Answer from the drawing. Dimensions are ordinates in mm from the lowest x, y and z of the part. A direction names the side the tool comes from. Coordinates: 2 decimals unless noted, no trailing zeros. Write each loop counter-clockwise with the first axis right and the second up, starting at its lowest first coordinate (ties: lowest second). Pieces come first, ordered by that corner, then holes. Notation, with made-up numbers: (49, 33.25) -> (68, 33.25) arc R20 cw to (68, 49.25) -> close; hole circle Ø1 at (54.25, -31.5). An arc over 180 degrees is marked (long way). Answer as a JSON object with one key per item and string values. Group by question number.
(1) Find section D-D (y = 4.5). Give the vertices of the cut face in (x, z).
(2) Flat-ended cylindrical pins translate along their axes: P1, Ø3, axis at y = 11.5, z = 4.5, coming from the -X side; P2, Ø1.5, axis at x = 16.5, z = 0.5, coming from the +Y side; P3, Ø1.2, axis at x = 17.5, z = 3, coming from the -Y side. Find the tip coordinate at first contact, or state that the pin passes through.
(3) For a pull along X with two mould halves and no side action, classify the marked faces 3, 4, 5 and 6 as +X half, -X half, draft (parallel to the pull), parting line (faces both ways), or undercut.
(4) Find section B-B (y = 10). Give the vertices of the cut face in (x, z) (1 decimal).
(5) Straight lines are drawn through the part: L1, parallel to Y at x = 10.5, z = 2.7; L2, parallel to X at y = 1.9, z = 2.95; L3, parallel to X at y = 10.75, z = 2. For each, find the intervals that lie inside material, in ascending order.
(6) Find section A-A (z = 0.9). Give the vertices of the cut face in (x, y).
(7) Find section C-C (x = 16.5). Give the vertices of the cut face in (y, z).
(8) Which of the six approach directions +Z, -Z, +X, -X, +Y, -Y give full straight-line access (tool end or side, diameter ignored) to the marked faces 1 and 2?
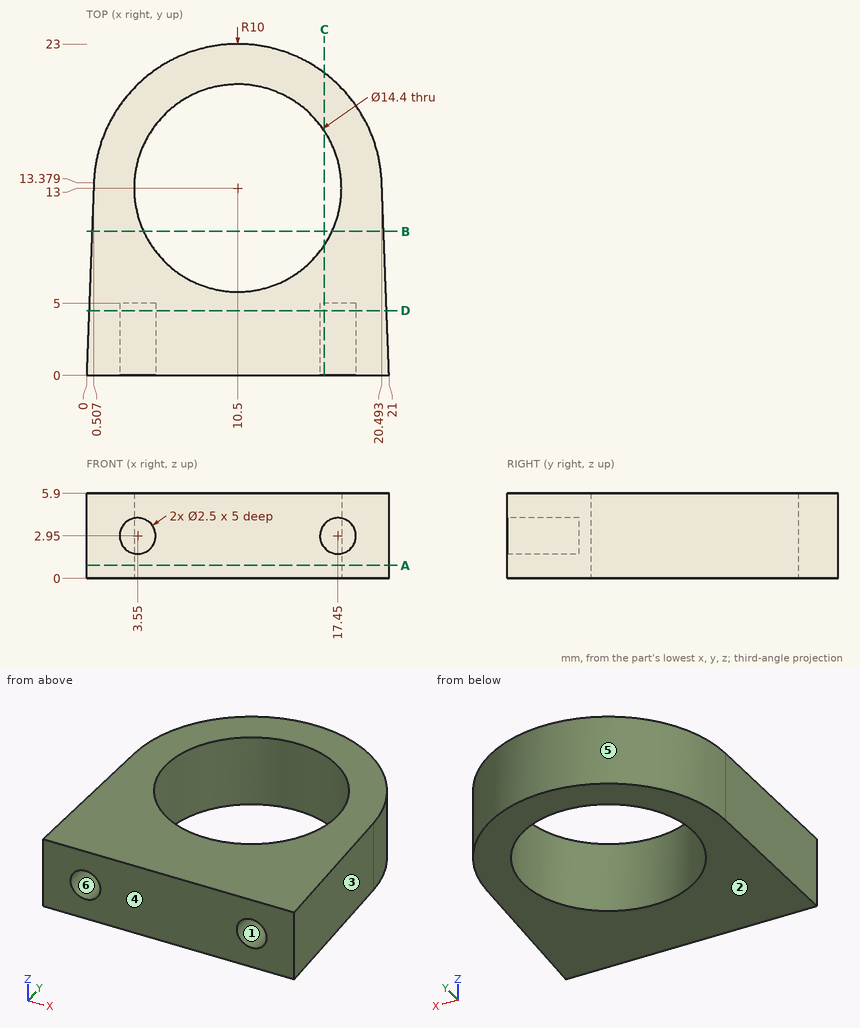
Results below:
{
 "1": {"outline": "(0.17, 0) -> (20.83, 0) -> (20.83, 5.9) -> (0.17, 5.9) -> close; hole circle Ø2.5 at (3.55, 2.95); hole circle Ø2.5 at (17.45, 2.95)"},
 "2": {"P1": "stops at x = 0.38", "P2": "stops at y = 21.51", "P3": "stops at y = 5"},
 "3": {"face 3": "+X half", "face 4": "draft", "face 5": "parting line", "face 6": "undercut"},
 "4": {"outline": "(0.4, 0) -> (4, 0) -> (4, 5.9) -> (0.4, 5.9) -> close; (17, 0) -> (20.6, 0) -> (20.6, 5.9) -> (17, 5.9) -> close"},
 "5": {"L1": "y = 0 to 5.8, 20.2 to 23", "L2": "x = 0.07 to 2.3, 4.8 to 16.2, 18.7 to 20.93", "L3": "x = 0.41 to 3.66, 17.34 to 20.59"},
 "6": {"outline": "(0, 0) -> (21, 0) -> (20.49, 13.38) arc R10 ccw to (0.51, 13.38) -> close; hole circle Ø14.4 at (10.5, 13)"},
 "7": {"outline": "(0, 0) -> (9.02, 0) -> (9.02, 5.9) -> (0, 5.9) -> (0, 3.76) -> (5, 3.76) -> (5, 2.14) -> (0, 2.14) -> close; (16.98, 0) -> (21, 0) -> (21, 5.9) -> (16.98, 5.9) -> close"},
 "8": {"face 1": "-Y", "face 2": "-Z, +X, -X, +Y, -Y"}
}
